```python
from build123d import *

# Parameters (mm, degrees)
ESQUISSE2_R                  = 76
ESQUISSE2_R_2                = 74
BOSS_EXTRU_1_DEPTH           = 138
ENL_V_MAT_EXTRU_1_DEPTH      = 649.747842898
ENL_V_MAT_EXTRU_1_DEPTH_BACK = 649.747842898
ESQUISSE3_R                  = 2.5


with BuildPart() as part:
    # Esquisse1 → Révolution3 (revolve)
    with BuildSketch(Plane.XY, mode=Mode.PRIVATE) as r_volution3_sk:
        with BuildLine():
            Line((-501.300996115, 74), (-500.300996115, 74))
            add(Edge.make_bspline(
                [(-500.300996115, 74), (-205.033047174, 74), (91.764741907, 0)],
                knots=[0, 0, 0, 1, 1, 1], degree=2))
            Line((91.764741907, 0), (108.299003885, 0))
            Line((108.299003885, 0), (92.73242949, 3.881182905))
            add(Edge.make_bspline(
                [(-500.300996115, 78), (-475.642620813, 78), (-426.347775001, 77.227857011), (-327.655384553, 72.595044211), (-228.880403388, 63.329565703), (-130.008955254, 49.431853826), (-68.17659714, 38.81586159), (-18.687478169, 29.165105527), (18.439887897, 21.348330719), (49.391507437, 14.351271458), (74.152443409, 8.465691784), (86.545764546, 5.42369172), (92.73242949, 3.881182905)],
                knots=[0, 0, 0, 0, 0.125, 0.25, 0.5, 0.625, 0.75, 0.8125, 0.875, 0.9375, 0.96875, 1, 1, 1, 1], degree=3))
            Line((-500.300996115, 78), (-501.300996115, 78))
            Line((-501.300996115, 78), (-501.300996115, 74))
        make_face()
    revolve(r_volution3_sk.sketch.rotate(Axis((-218.288054544, 0, 0), (1, 0, 0)), 90), axis=Axis((-218.288054544, 0, 0), (1, 0, 0)))

    # Esquisse2 → Boss.-Extru.1 (add)
    with BuildSketch(Plane.ZY.offset(501.300996115)):
        with Locations(Location((0, 0, 0), (0, 0, 180))):
            Circle(ESQUISSE2_R)
        Circle(ESQUISSE2_R_2, mode=Mode.SUBTRACT)
    extrude(amount=BOSS_EXTRU_1_DEPTH)

    # Esquisse3 → Enlèv. mat.-Extru.1 (cut, two sides: drawn at the far end of the back side and taken through both)
    with BuildSketch(Plane(origin=(0, 0, 0), x_dir=(1, 0, 0), z_dir=(0, 1, 0)).offset(-ENL_V_MAT_EXTRU_1_DEPTH_BACK)):
        with Locations(Location((-496.300996115, 0, 0), (0, 0, 270))):
            Circle(ESQUISSE3_R)
    extrude(amount=ENL_V_MAT_EXTRU_1_DEPTH + ENL_V_MAT_EXTRU_1_DEPTH_BACK, mode=Mode.SUBTRACT)


solid = part.part
```
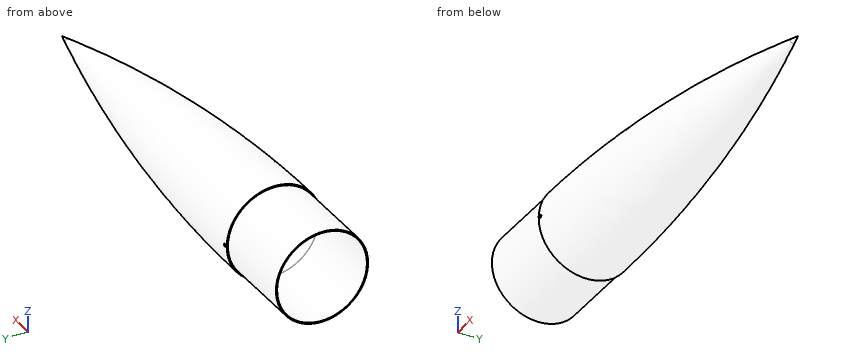
Source: CAD feature listing. Evaluate the final solid. Frame: model axes, mm. Coordinates: 2 decimals unless noted, no trailing zeros. Loops run counter-clockwise (first coordinate to the right, second up) from the corner with the lowest first, then second, coordinate; pieces in that order, holes last. Notation, with made-up numbers: (69, 44) -> (78, 44) arc R26 cw to (78, 60) -> close; hole circle Ø6 at (83.5, 5.5). An arc over 180 degrees is marked (long way). One line per item, written item: value. Start each with the question number.
Q1. Contact query for flat-ended pins moving along their axis: P1, Ø6, axis at x = -170.5, y = -12.5, coming from the -Z side; P2, Ø4, axis at x = -75, z = 1, coming from the -Y side; P3, Ø3, axis at x = -496.3, z = 0, coming from the -Y side; P4, Ø2, axis at x = -23.5, z = 10, coming from the -Y side. Output: stop coordinate, or through.
Q2. Line query: line 1 along Y through (x, z) = (-500.95, 0); line 2 along Y through (x, z) = (-530, 0); line 3 along Z through (x, y) = (-587, -47.5). Output: solid intervals per line, ascending.
Q3. Section query A-A, the plane x = -547. Return the cut outline in (y, z), and give its area (3 significant figures).
Results:
1. P1: z = -54.34
1. P2: y = -40.17
1. P3: through
1. P4: y = -28.72
2. line 1: -78 to -74, 74 to 78
2. line 2: -76 to -74, 74 to 76
2. line 3: -59.33 to -56.74, 56.74 to 59.33
3. outline: circle Ø152 at (0, 0); hole circle Ø148 at (0, 0)
3. area: 942 mm^2
